The drawing under review shows one solid part. Ordinate dimensions are in mm from its lowest x, y, z. Give positions to 0.01 mm unless a question says otherwise; leave off trailing zeros. Loops run counter-clockwise (first coordinate to the right, second up) from the corner with the lowest first, then second, coordinate; pieces in that order, holes last. Notation, with made-up numbers: (53, 28.5) - (97, 28.5) arc R20 cw to (97, 54.5) - close; hole circle Ø9 at (6.5, 9.5). An arc over 180 degrees is marked (long way). Write each question's results on one line, items separated by ' | '.
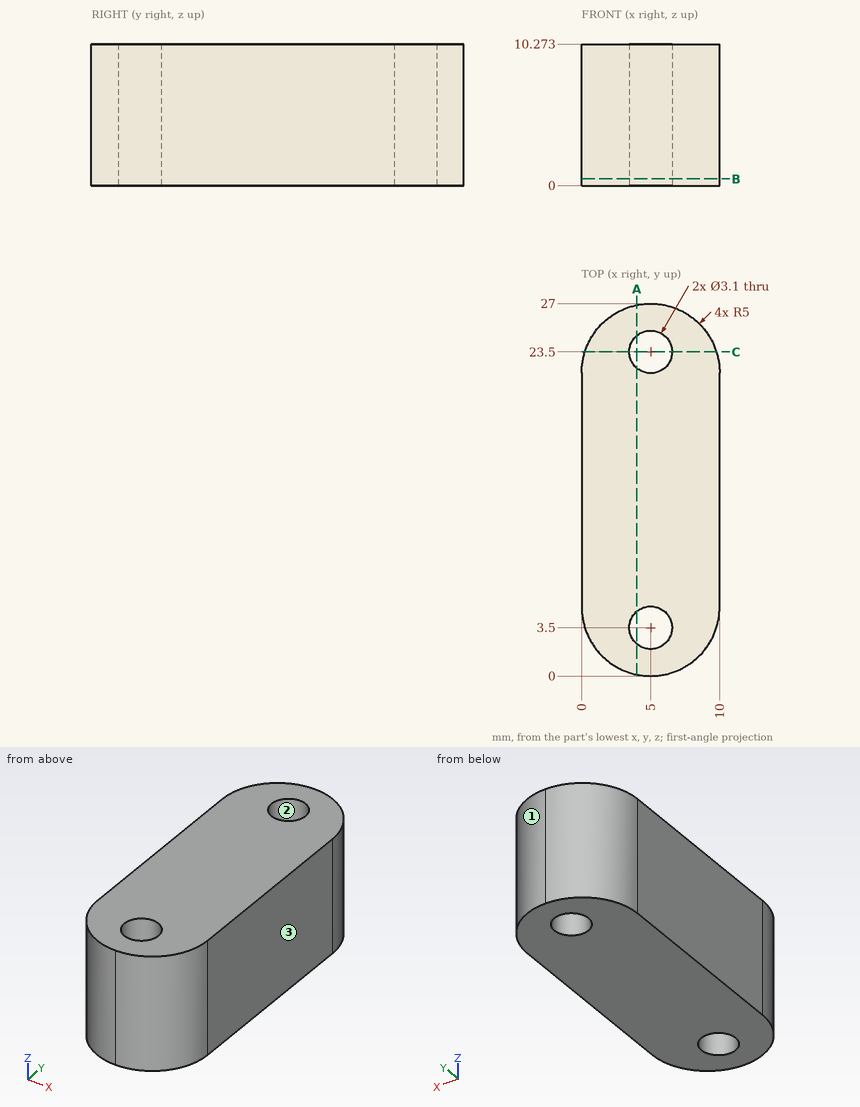
(1) Wall thickness on line 1 along Y through (x, z) = (5, 3.25); line 2 along Y through (x, z) = (4, 1) (1 decimal); line 3 along X through (y, z) = (23.5, 3.5): over which ranges is each line inside the solid? List them lowest first. Write a range as from..to.
Answers below:
line 1: 0..1.95, 5.05..21.95, 25.05..27 | line 2: 0.1..2.3, 4.7..22.3, 24.7..26.9 | line 3: 0.23..3.45, 6.55..9.77
(2) Insertion check: P1, Ø2.5, axis at x = 5, y = 23.5, coming from the +Z side; P2, Ø2, axis at x = 8, y = 9, coming from the -Z side; P3, Ø2, axis at x = 2.5, z = 7, coming from the -Y side. Each pin has a flat end and moves straight along its axis. Give the tip position at first contact, or say it passes through.
Answers below:
P1: through | P2: z = 0 | P3: y = 0.23
(3) Draft analysis for pull direction Y (two halves, no side actions). For the marked faces 1, 2 and 3, state which applies: pulls with the +Y half, pulls with the -Y half, needs draft (parallel to the pull), parting line crosses it, or undercut.
Answers below:
face 1: pulls with the +Y half | face 2: undercut | face 3: needs draft
(4) Take a section at A-A on x = 4. Give the boundary of the cut face in (y, z) (1 decimal).
Answers below:
outline: (0.1, 0) - (2.3, 0) - (2.3, 10.3) - (0.1, 10.3) - close; (4.7, 0) - (22.3, 0) - (22.3, 10.3) - (4.7, 10.3) - close; (24.7, 0) - (26.9, 0) - (26.9, 10.3) - (24.7, 10.3) - close
(5) Take a section at B-B on z = 0.5. Count the separate pieces of the cut face and the enclosed holes in it.
Answers below:
separate pieces: 1 | enclosed holes: 2
(6) Take a section at C-C on y = 23.5. Give the boundary of the cut face in (x, z).
Answers below:
outline: (0.23, 0) - (3.45, 0) - (3.45, 10.27) - (0.23, 10.27) - close; (6.55, 0) - (9.77, 0) - (9.77, 10.27) - (6.55, 10.27) - close
